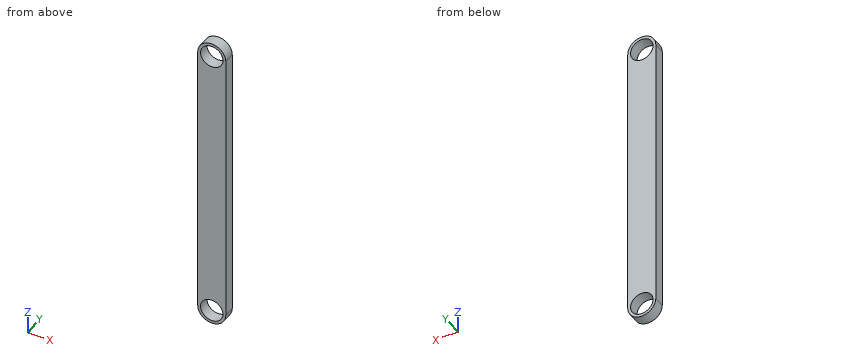
from build123d import *

# Parameters (mm, degrees)
F0_R     = 5.08
F1_DEPTH = 5.08


with BuildPart() as f1:
    # F0 (on Front) → F1 (new body)
    with BuildSketch(Plane.XZ):
        with BuildLine():
            Line((6.35, -46.644763), (6.35, 80.355237))
            ThreePointArc((6.35, 80.355237), (0, 74.005237), (-6.35, 80.355237))
            Line((-6.35, 80.355237), (-6.35, -46.644763))
            ThreePointArc((-6.35, -46.644763), (0, -40.294763), (6.35, -46.644763))
        make_face()
        with BuildLine():
            ThreePointArc((-6.35, 80.355237), (0, 74.005237), (6.35, 80.355237))
            ThreePointArc((6.35, 80.355237), (0, 86.705237), (-6.35, 80.355237))
        make_face()
        with Locations((0, 80.355237)):
            Circle(F0_R, mode=Mode.SUBTRACT)
        with BuildLine():
            ThreePointArc((-6.35, -46.644763), (0, -52.994763), (6.35, -46.644763))
            ThreePointArc((6.35, -46.644763), (0, -40.294763), (-6.35, -46.644763))
        make_face()
        with Locations((0, -46.644763)):
            Circle(F0_R, mode=Mode.SUBTRACT)
    extrude(amount=F1_DEPTH)


solid = f1.part
Read the model definition and answer for the solid it produces. Units are mm, in the model's axes. Give positions to 0.01 mm unless a question says otherwise; leave off trailing zeros. Write each loop counter-clockwise with the first axis right and the second up, starting at its lowest first coordinate (ties: lowest second). Pieces come first, ordered by that corner, then holes. Notation, with made-up numbers: (8, -26.75) - (22, -26.75) arc R9 cw to (22, -22.75) - close; hole circle Ø8 at (-31.75, 14.25). An arc over 180 degrees is marked (long way). Use CSV: the item, a comma, the result in double quotes. Start each with the question number.
(1) Given P1, Ø2, axis at x = -3.5, y = -1, coming from the +Z side; P2, Ø3, axis at x = -2, y = -2, coming from the +Z side, each flat-ended and moving along its own axis, determine where each tip first touches the part or whether it passes through.
(2) Find section A-A (x = 0). Give the vertices of the cut face in (y, z), plus the area to 3 significant figures.
(3) Consider line 1 along Z through (x, y) = (0, -3.15); line 2 along Z through (x, y) = (3.25, -1.6); line 3 along X through (y, z) = (-3.8, 78). Determine where each line is inside the solid, lowest interval first.
(4) Find section B-B (y = -1.9). Give the vertices of the cut face in (x, z).
Findings below:
1,P1,"z = 86.19"
1,P2,"z = 86.69"
2,outline,"(-5.08, -52.99) - (0, -52.99) - (0, -51.72) - (-5.08, -51.72) - close; (-5.08, -41.56) - (0, -41.56) - (0, 75.28) - (-5.08, 75.28) - close; (-5.08, 85.44) - (0, 85.44) - (0, 86.71) - (-5.08, 86.71) - close"
2,area,"606 mm2"
3,line 1,"-52.99 to -51.72, -41.56 to 75.28, 85.44 to 86.71"
3,line 2,"-52.1 to -50.55, -42.74 to 76.45, 84.26 to 85.81"
3,line 3,"-6.35 to -4.5, 4.5 to 6.35"
4,outline,"(-6.35, -46.64) arc R6.35 ccw to (6.35, -46.64) - (6.35, 80.36) arc R6.35 ccw to (-6.35, 80.36) - close; hole circle Ø10.16 at (0, -46.64); hole circle Ø10.16 at (0, 80.36)"
